Work out the finished part from the listing and answer in its coordinate system (mm). A direction names the side the tool comes from. Give positions to 0.01 mm unless a question says otherwise; leave off trailing zeros. Order: outer loops, then holes, each group sorted by start corner. A loop starts at its lowest first (then second) coordinate and runs counter-clockwise, first axis right, second up.
```python
from build123d import *

# Parameters (mm, degrees)
F0_R     = 29.75
F0_R_2   = 28.25
F1_DEPTH = 3
F2_DEPTH = 0.5
F3_R     = 1


with BuildPart() as f1:
    # F0 (on Top) → F1 (new body)
    with BuildSketch(Plane.XY):
        Circle(F0_R)
        Circle(F0_R_2, mode=Mode.SUBTRACT)
    extrude(amount=F1_DEPTH)

    # F0 (on Top) → F2 (join)
    with BuildSketch(Plane.XY):
        Circle(F0_R)
        Circle(F0_R_2, mode=Mode.SUBTRACT)
        Circle(F0_R_2)
    extrude(amount=F2_DEPTH)

    # F3
    f3_edges = [f1.edges().sort_by_distance(p)[0] for p in [
        (-28.25, 0, 3),
        (-28.25, 0, 0.5),
    ]]
    fillet(f3_edges, radius=F3_R)


solid = f1.part
```
1. The mould has two halves that part along X. Classify faces 3 (the face through (15.993, 25.085, 1.479)), 4 (the face through (15.19, 23.82, 1.75)), 5 (the face through (21.9, -19.7, 3)): pulls with the +X half, pulls with the -X half, needs draft (parallel to the pull), parting line crosses it, or undercut.
Findings below:
face 3: parting line crosses it
face 4: undercut
face 5: needs draft
2. Straight lines are drawn through the part: probe 1 along Y at (x, z) = (0, 1.65); probe 2 along Z at (x, y) = (-10, 15.5); probe 3 along Y at (x, z) = (-16, 1.35). For each, find the intervals that lie inside material, in ascending order.
Findings below:
probe 1: y = -29.75 to -28.25, 28.25 to 29.75
probe 2: z = 0 to 0.5
probe 3: y = -25.08 to -23.27, 23.27 to 25.08
3. Which of the six approach directions +Z, -Z, +X, -X, +Y, -Y give full straight-line access (tool end or side, diameter ignored) to faces 1 (the face through (0, 0, 0)), 2 (the face through (0, 0, 0.5))?
Findings below:
face 1: -Z, +X, -X, +Y, -Y
face 2: +Z
4. The part is cut by section A-A (y = 0). Write down the section's boundary in (x, z).
Findings below:
outline: (-29.75, 0) - (29.75, 0) - (29.75, 3) - (29.25, 3) arc R1 ccw to (28.25, 2) - (28.25, 1.5) arc R1 cw to (27.25, 0.5) - (-27.25, 0.5) arc R1 cw to (-28.25, 1.5) - (-28.25, 2) arc R1 ccw to (-29.25, 3) - (-29.75, 3) - close
5. Given P1, Ø1, axis at y = 18, z = 2, coming from the +X side; P2, Ø10, axis at x = 6.5, y = -9, coming from the +Z side, each flat-ended and moving along its own axis, determine where each tip first touches the part or whether it passes through.
Findings below:
P1: stops at x = 24.06
P2: stops at z = 0.5
